Here's the drawing with two shaded views (mm, measured from the low corner). I have some questions. A direction names the side the tool comes from. Coordinates: 2 decimals unless noted, no trailing zeros. Write each loop counter-clockwise with the first axis right and the second up, starting at its lowest first coordinate (ties: lowest second). Pieces come first, ordered by that corner, then holes.
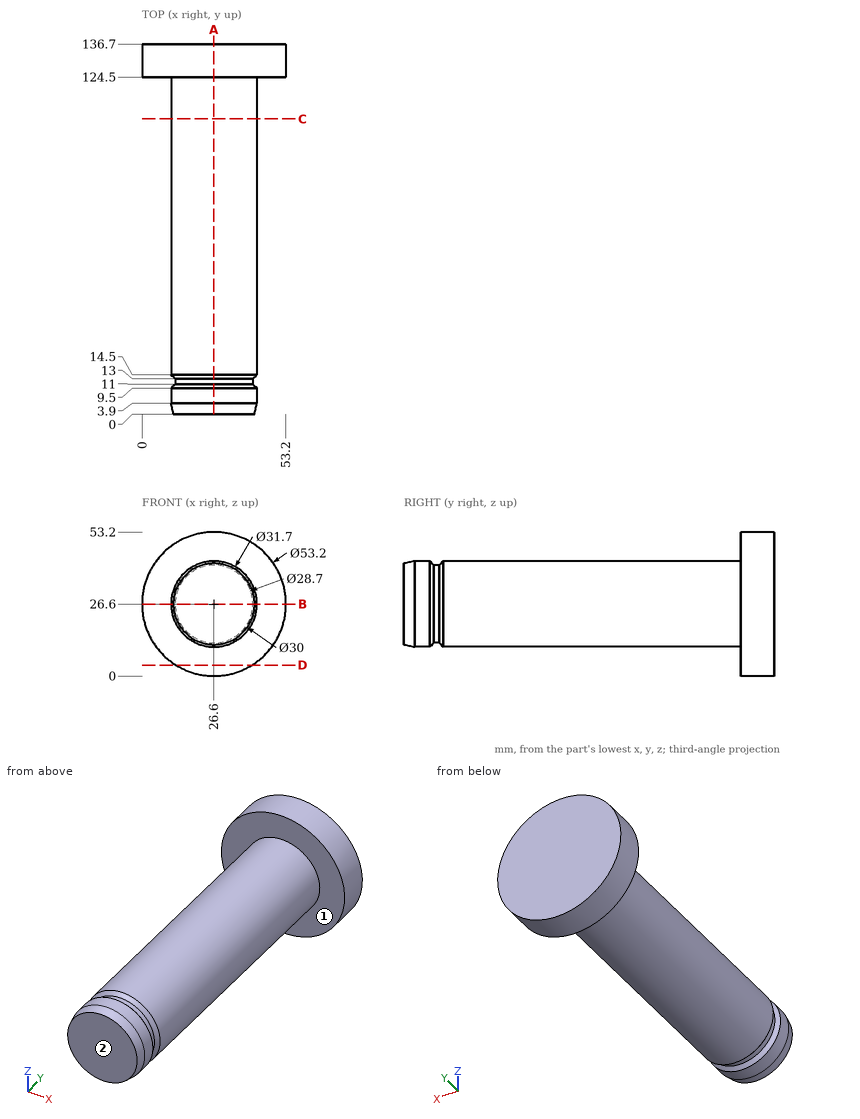
1. If we section it at B-B, the plane z = 26.6: List the corners of the cut face in (x, y) for me, plus the area to 3 significant figures.
2. I'm going to push flat-ended pins straight in: P1, Ø3, axis at x = 37.5, y = 68, coming from the -Z side; P2, Ø8, axis at y = 104.5, z = 47, coming from the -X side; P3, Ø2, axis at x = 18, y = 23.5, coming from the +Z side; P4, Ø16, axis at x = 15.5, z = 14, coming from the -Y side. Where does each tip first touch, or does it pass through?
3. If we section it at A-A, the plane x = 26.6: List the corners of the cut face in (y, z) for me.
4. If I drill on L1, parallel to Z at x = 26, y = 121.5; L2, parallel to Y at x = 44, z = 9.5; L3, parallel to X at y = 126.5, z = 11, over which ranges is the centre line in solid material (lowest first)?
5. Which directions (+Z, -Z, +X, -X, +Y, -Y) give clear straight access to the entire face, cutting with the end or side of a thin tool? Please do the marked faces 1 and 2.
6. If we section it at D-D, the plane z = 4: List the corners of the cut face in (x, y) for me.
7. If we section it at C-C, the plane y = 109: List the corners of the cut face in (x, z) for me.
Answers:
1. outline: (0, 124.5) - (10.75, 124.5) - (10.75, 14.5) - (12.25, 13) - (12.25, 11) - (10.75, 9.5) - (10.75, 3.9) - (11.6, 0) - (41.6, 0) - (42.45, 3.9) - (42.45, 9.5) - (40.95, 11) - (40.95, 13) - (42.45, 14.5) - (42.45, 124.5) - (53.2, 124.5) - (53.2, 136.7) - (0, 136.7) - close
1. area: 4,580 mm2
2. P1: stops at z = 13.84
2. P2: passes through
2. P3: stops at z = 40.51
2. P4: stops at y = 0
3. outline: (0, 11.6) - (3.9, 10.75) - (9.5, 10.75) - (11, 12.25) - (13, 12.25) - (14.5, 10.75) - (124.5, 10.75) - (124.5, 0) - (136.7, 0) - (136.7, 53.2) - (124.5, 53.2) - (124.5, 42.45) - (14.5, 42.45) - (13, 40.95) - (11, 40.95) - (9.5, 42.45) - (3.9, 42.45) - (0, 41.6) - close
4. L1: z = 10.76 to 42.44
4. L2: y = 124.5 to 136.7
4. L3: x = 5.05 to 48.15
5. face 1: -Y
5. face 2: +Z, -Z, +X, -X, -Y
6. outline: (12.57, 124.5) - (40.63, 124.5) - (40.63, 136.7) - (12.57, 136.7) - close
7. outline: circle Ø31.7 at (26.6, 26.6)
